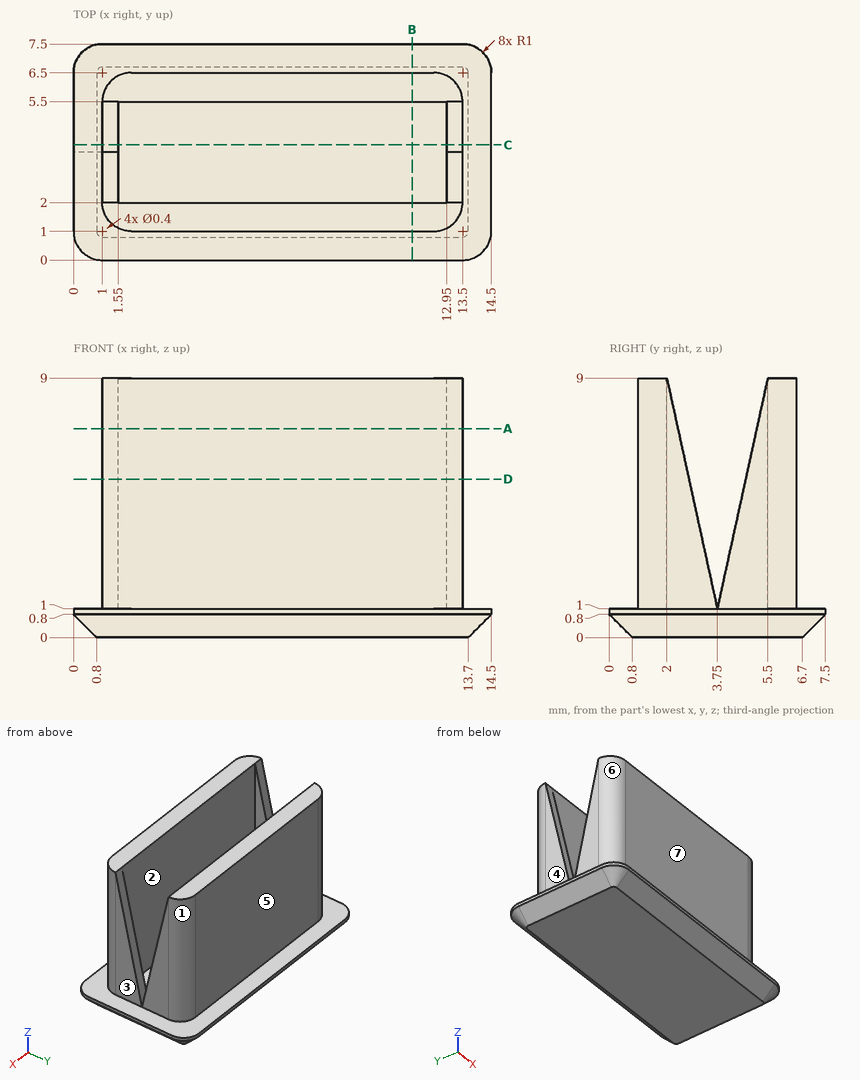
Study the drawing (mm; zero at the part's minimum x, y, z) and answer. A direction names the side the tool comes from. Give positions to 0.01 mm unless a question says otherwise; leave off trailing zeros. Write each loop counter-clockwise with the first axis right and the second up, starting at its lowest first coordinate (ties: lowest second). Pieces come first, ordered by that corner, then holes. Notation, with made-up numbers: (42.25, 5.5) -> (76.25, 5.5) arc R16 ccw to (76.25, 12.5) -> close; hole circle Ø1 at (12.5, 12). An arc over 180 degrees is marked (long way). Write item = value, one per line. Start each with the question number.
1) The part is cut by section D-D, the plane z = 5.5. Determine the outline of the cut face in (x, y).
2) Determine the mould class of the marked faces 1, 2 and 3 for opening direction Y: +Y half, -Y half, draft (parallel to the pull), parting line (faces both ways), or undercut.
3) The part is cut by section A-A, the plane z = 7.25. Determine the outline of the cut face in (x, y).
4) Straight lines are drawn through the part: line 1 along Y through (x, z) = (5.5, 6); line 2 along X through (y, z) = (2.5, 3.75); line 3 along Z through (x, y) = (1, 1). For each, find the intervals that lie inside material, in ascending order.
5) The part is cut by section C-C, the plane y = 4. Determine the outline of the cut face in (x, z), and give its area (3 significant figures).
6) Each of these flat-tipped pins is pushed along its axis until it touches: pin 1 (0.5 mm diameter, centred on y = 4.5, z = 5, fed in from -X); pin 2 (5 mm diameter, centred on x = 11.5, z = 4.5, fed in from +Y); pin 3 (3 mm diameter, centred on x = 6.5, z = 6, fed in from -Y). Where does it stop, or does it pass through?
7) Which of the six approach directions +Z, -Z, +X, -X, +Y, -Y give full straight-line access (tool end or side, diameter ignored) to the marked faces 4, 5, 6 and 7?
8) The part is cut by section B-B, the plane x = 11.75. Determine the outline of the cut face in (y, z).
Solutions:
q1.outline = (1, 2) arc R1 ccw to (2, 1) -> (12.5, 1) arc R1 ccw to (13.5, 2) -> (13.5, 2.77) -> (12.95, 2.77) -> (12.95, 2) -> (1.55, 2) -> (1.55, 2.77) -> (1, 2.77) -> close; (1, 4.73) -> (1.55, 4.73) -> (1.55, 5.5) -> (12.95, 5.5) -> (12.95, 4.73) -> (13.5, 4.73) -> (13.5, 5.5) arc R1 ccw to (12.5, 6.5) -> (2, 6.5) arc R1 ccw to (1, 5.5) -> close
q2.face_1 = +Y half
q2.face_2 = undercut
q2.face_3 = draft
q3.outline = (1, 2) arc R1 ccw to (2, 1) -> (12.5, 1) arc R1 ccw to (13.5, 2) -> (13.5, 2.38) -> (12.95, 2.38) -> (12.95, 2) -> (1.55, 2) -> (1.55, 2.38) -> (1, 2.38) -> close; (1, 5.12) -> (1.55, 5.12) -> (1.55, 5.5) -> (12.95, 5.5) -> (12.95, 5.12) -> (13.5, 5.12) -> (13.5, 5.5) arc R1 ccw to (12.5, 6.5) -> (2, 6.5) arc R1 ccw to (1, 5.5) -> close
q4.line_1 = 1 to 2, 5.5 to 6.5
q4.line_2 = 1 to 1.55, 12.95 to 13.5
q4.line_3 = 0 to 1
q5.outline = (0, 0.8) -> (0.8, 0) -> (13.7, 0) -> (14.5, 0.8) -> (14.5, 1) -> (13.5, 1) -> (13.5, 2.14) -> (12.95, 2.14) -> (12.95, 1) -> (1.55, 1) -> (1.55, 2.14) -> (1, 2.14) -> (1, 1) -> (0, 1) -> close
q5.area = 15.1 mm²
q6.pin_1 = 1
q6.pin_2 = 6.5
q6.pin_3 = 1
q7.face_4 = +Z, -X, +Y, -Y
q7.face_5 = +Z, +X, -X, +Y
q7.face_6 = +Z, -X, -Y
q7.face_7 = +Z, +X, -X, -Y
q8.outline = (0, 0.8) -> (0.8, 0) -> (6.7, 0) -> (7.5, 0.8) -> (7.5, 1) -> (6.5, 1) -> (6.5, 9) -> (5.5, 9) -> (5.5, 1) -> (2, 1) -> (2, 9) -> (1, 9) -> (1, 1) -> (0, 1) -> close
